The listing builds one solid part. Answer for the finished solid, in the listing's coordinates (mm). Give positions to 0.01 mm unless a question says otherwise; leave off trailing zeros. Write each loop counter-clockwise with the first axis right and the second up, starting at its lowest first coordinate (ties: lowest second). Pieces come first, ordered by that corner, then holes. Notation, with made-up numbers: M -37.5,-10 L 12.5,-10 A9 ccw 12.5,-5 Z; hole C 66.25,-22.75 d5. An arc over 180 degrees is marked long. Answer as a JSON object with one key per item and string values.
```python
from build123d import *

# Parameters (mm, degrees)
SWEEP1_PROFILE_R     = 12.7
CUT_SWEEP1_PROFILE_R = 9.525
SKETCH19_R           = 6.35
BOSS_EXTRUDE1_DEPTH  = 76.2
SKETCH28_R           = 3.175
BOSS_EXTRUDE2_DEPTH  = 50.8


with BuildPart() as part:
    # Sweep1: sweep along a path in Sketch2
    with BuildLine(Plane(origin=(0, 0, 0), x_dir=(0, 0, -1), z_dir=(1, 0, 0))) as sweep1_path:
        Line((-248.182278836, -217.015933946), (-32.65613193, -1.489787041))
        Line((-32.65613193, -1.489787041), (272.14386807, -1.489787041))
        Line((272.14386807, -1.489787041), (487.670014975, -217.015933946))
    # Sweep1 profile (on start of the path) → Sweep1 (sweep)
    with BuildSketch(Plane(origin=(0, -217.015933946, 248.182278836), x_dir=(0, 0.707106781, 0.707106781), z_dir=(0, 0.707106781, -0.707106781))):
        Circle(SWEEP1_PROFILE_R)
    sweep(path=sweep1_path.line, transition=Transition.RIGHT)

    # Cut-Sweep1: sweep along a path in Sketch2_2
    with BuildLine(Plane(origin=(0, 0, 0), x_dir=(0, 0, -1), z_dir=(1, 0, 0))) as cut_sweep1_path:
        Line((-248.182278836, -217.015933946), (-32.65613193, -1.489787041))
        Line((-32.65613193, -1.489787041), (272.14386807, -1.489787041))
        Line((272.14386807, -1.489787041), (487.670014975, -217.015933946))
    # Cut-Sweep1 profile (on start of the path) → Cut-Sweep1 (sweep, cut)
    with BuildSketch(Plane(origin=(0, -217.015933946, 248.182278836), x_dir=(0, 0.707106781, 0.707106781), z_dir=(0, 0.707106781, -0.707106781))):
        Circle(CUT_SWEEP1_PROFILE_R)
    sweep(path=cut_sweep1_path.line, transition=Transition.RIGHT, mode=Mode.SUBTRACT)

    # Sketch19 → Boss-Extrude1 (add)
    with BuildSketch(Plane(origin=(0, 0, 0), x_dir=(0, 0, -1), z_dir=(1, 0, 0))):
        with Locations((119.74386807, -1.489787041)):
            Circle(SKETCH19_R)
    extrude(amount=BOSS_EXTRUDE1_DEPTH)

    # Sketch28 → Boss-Extrude2 (add)
    with BuildSketch(Plane(origin=(0, 0, 0), x_dir=(0, 0, -1), z_dir=(1, 0, 0))):
        with Locations((377.089758854, -106.435677825)):
            Circle(SKETCH28_R)
    extrude(amount=BOSS_EXTRUDE2_DEPTH)


solid = part.part
```
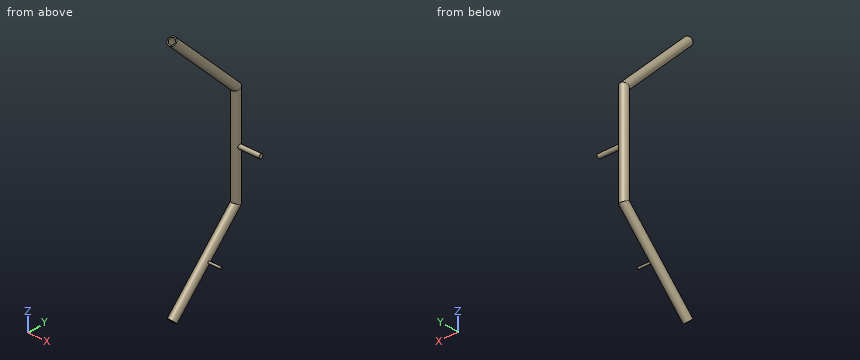
1. Flat-ended cylindrical pins translate along their axes: pin 1 (5 mm diameter, centred on y = -107.5, z = -376.5, fed in from +X); pin 2 (1.5 mm diameter, centred on x = 30.5, z = -111, fed in from -Y); pin 3 (5 mm diameter, centred on x = -1, z = 139.5, fed in from -Y); pin 4 (22 mm diameter, centred on x = 0, y = -1.49, fed in from +Z). Find the tip coordinate at first contact, or state that the pin passes through.
Verdict:
{"pin 1": "stops at x = 50.8", "pin 2": "passes through", "pin 3": "stops at y = -128.75", "pin 4": "stops at z = 61.62"}
2. Consider line 1 along Z through (x, y) = (3, -18); line 2 along Z through (x, y) = (-4, -110); line 3 along Y through (x, z) = (8, -410). Determine where each line is inside the solid, lowest interval first.
Verdict:
{"line 1": "z = -306.11 to -301.44, -275.87 to -271.2, 31.71 to 36.38, 61.95 to 66.62", "line 2": "z = -397.7 to -392.88, -368.43 to -363.61, 124.12 to 128.94, 153.39 to 158.21", "line 3": "y = -153.3 to -146.66, -132.03 to -125.4"}
3. A cutting plane is placed at A-A, the plane z = 4. Give the vertices of the cut face in (x, y) (3 decimals).
Verdict:
{"outline": "C 0,-1.49 d25.4; hole C 0,-1.49 d19.05"}
4. A cutting plane is placed at B-B, the plane y = -31.5. Count the separate pieces of the cut face and the enclosed holes in it, plus the area to 3 significant figures.
Verdict:
{"separate pieces": "2", "enclosed holes": "2", "area": "627 mm2"}
